Verification items for the finished model (mm, model axes). A direction names the side the tool comes from. Give positions to 0.01 mm unless a question says otherwise; leave off trailing zeros. Write each loop counter-clockwise with the first axis right and the second up, starting at its lowest first coordinate (ties: lowest second). Pieces come first, ordered by that corner, then holes. Notation, with made-up numbers: (2, 10) - (8, 10) arc R26 ccw to (8, 35) - close; hole circle Ø11 at (68, 42). An arc over 180 degrees is marked (long way). Answer as a JSON object with one key per item and string values. Group by question number.
Item 1: Draft check along Z on faces 3 (the face through (23.846, 1.521, -7.509)), 4 (the face through (0, 23.712, 9)), 5 (the face through (10.25, 12, 0)). Enter one of: +Z half, -Z half, draft (parallel to the pull), parting line (faces both ways), or undercut.
Item 2: Tool access check on faces 1 (the face through (0, 0, 0)), 2 (the face through (10.99, 22.95, 0.09)). Record the directions out of +Z, -Z, +X, -X, +Y, -Y that give a thin tool (end or side, any length) a straight path to the whole face; none if there is none.
Item 3: Sectioned sample at C-C, the plane y = 12.75. Record the boundary of the cut face in (x, z).
Item 4: Sectioned sample at A-A, the plane z = 0. Record the boundary of the cut face in (x, y).
Item 5: Sectioned sample at B-B, the plane x = 0. Record the boundary of the cut face in (y, z), and give its area (3 significant figures).
Item 6: Scan lines: line 1 along Z through (x, y) = (0, 21.5); line 2 along Z through (x, y) = (4.5, 12.5); line 3 along X through (y, z) = (10.75, 8). Record each from-to range of solid material in increasing order. Write a range as [from, to].
Item 7: Sectioned sample at D-D, the plane y = 17.75. Record the boundary of the cut face in (x, z), and give its area (3 significant figures).
Item 8: Go/stop test with flat-tipped pins: pin 1 (1.5 mm diameter, centred on y = 10.5, z = -7, fed in from +X); pin 2 (12 mm diameter, centred on y = 16.5, z = 12.5, fed in from +X); pin 3 (5 mm diameter, centred on y = 9.5, z = -2, fed in from -X). Record where each tip stops, or that it passes through.
```python
from build123d import *

# Parameters (mm, degrees)
SKETCH001_W  = 20.5
SKETCH001_H  = 10
POCKET_DEPTH = 21.713315
CHAMFER_SIZE = 1.5


with BuildPart() as part:
    # Sketch → Revolution (revolve)
    with BuildSketch(Plane.XY):
        with BuildLine():
            Line((0, 0), (25, 0))
            Line((25, 0), (25, 3))
            ThreePointArc((14, 23.712315), (16.920598, 11.986276), (25, 3))
            Line((14, 23.712315), (0, 23.712315))
            Line((0, 23.712315), (0, 0))
        make_face()
    revolve(axis=Axis((0, 0, 0), (0, 1, 0)))

    # Sketch001 → Pocket (cut, through all)
    with BuildSketch(Plane.XZ.offset(-2)):
        Rectangle(SKETCH001_W, SKETCH001_H)
    extrude(amount=-POCKET_DEPTH, mode=Mode.SUBTRACT)

    # Chamfer
    chamfer_edges = [part.edges().sort_by_distance(p)[0] for p in [
        (0, 23.712315, -5),
        (10.25, 23.712315, 0),
        (0, 23.712315, 5),
        (-10.25, 23.712315, 0),
    ]]
    chamfer(chamfer_edges, length=CHAMFER_SIZE)


solid = part.part
```
Geometry check:
{
 "1": {"face 3": "parting line", "face 4": "draft", "face 5": "undercut"},
 "2": {"face 1": "+Z, -Z, +X, -X, -Y", "face 2": "+Y"},
 "3": {"outline": "circle Ø33.06 at (0, 0); hole (-10.25, -5) - (10.25, -5) - (10.25, 5) - (-10.25, 5) - close"},
 "4": {"outline": "(-25, 0) - (25, 0) - (25, 3) arc R25 cw to (14, 23.71) - (11.75, 23.71) - (10.25, 22.21) - (10.25, 2) - (-10.25, 2) - (-10.25, 22.21) - (-11.75, 23.71) - (-14, 23.71) arc R25 cw to (-25, 3) - close"},
 "5": {"outline": "(0, -25) - (3, -25) arc R25 cw to (23.71, -14) - (23.71, -6.5) - (22.21, -5) - (2, -5) - (2, 5) - (22.21, 5) - (23.71, 6.5) - (23.71, 14) arc R25 cw to (3, 25) - (0, 25) - close", "area": "646 mm^2"},
 "6": {"line 1": "[-14.1, -5], [5, 14.1]", "line 2": "[-16.04, -5], [5, 16.04]", "line 3": "[-15.7, 15.7]"},
 "7": {"outline": "circle Ø29.44 at (0, 0); hole (-10.25, -5) - (10.25, -5) - (10.25, 5) - (-10.25, 5) - close", "area": "476 mm^2"},
 "8": {"pin 1": "x = 16.95", "pin 2": "x = 14.61", "pin 3": "x = -20.32"}
}
